The listing builds one solid part. Answer for the finished solid, in the listing's coordinates (mm). A direction names the side the tool comes from. Coordinates: 2 decimals unless noted, no trailing zeros. Write each loop counter-clockwise with the first axis right and the second up, starting at its lowest first coordinate (ties: lowest second). Pieces come first, ordered by that corner, then holes.
```python
from build123d import *

# Parameters (mm, degrees)
SKETCH1_W           = 30
SKETCH1_H           = 30
BOSS_EXTRUDE2_DEPTH = 35
SKETCH2_W           = 25
SKETCH2_H           = 25
CUT_EXTRUDE1_DEPTH  = 10
SKETCH3_R           = 5
SKETCH3_R_2         = 2
CUT_EXTRUDE4_DEPTH  = 20
SKETCH5_R           = 2
CUT_EXTRUDE5_DEPTH  = 25


with BuildPart() as part:
    # Sketch1 → Boss-Extrude2 (new body)
    with BuildSketch(Plane(origin=(0, 0, 0), x_dir=(1, 0, 0), z_dir=(0, 1, 0))):
        Rectangle(SKETCH1_W, SKETCH1_H)
    extrude(amount=BOSS_EXTRUDE2_DEPTH)

    # Sketch2 → Cut-Extrude1 (cut)
    with BuildSketch(Plane(origin=(0, 35, 0), x_dir=(1, 0, 0), z_dir=(0, 1, 0))):
        with Locations((2.5, 2.5)):
            Rectangle(SKETCH2_W, SKETCH2_H)
    extrude(amount=-CUT_EXTRUDE1_DEPTH, mode=Mode.SUBTRACT)

    # Sketch3 → Cut-Extrude4 (cut)
    # profile 1 of 2: a face of its own
    with BuildSketch(Plane(origin=(0, 25, 0), x_dir=(1, 0, 0), z_dir=(0, 1, 0))):
        with Locations(Location((-2.422862762, 7.422862762, 0), (0, 0, 270))):
            Circle(SKETCH3_R)
        with Locations(Location((-2.422862762, 7.422862762, 0), (0, 0, 270))):
            Circle(SKETCH3_R_2, mode=Mode.SUBTRACT)
    # profile 2 of 2: a face of its own
    with BuildSketch(Plane(origin=(0, 25, 0), x_dir=(1, 0, 0), z_dir=(0, 1, 0))):
        with Locations(Location((8.75, -3.75, 0), (0, 0, 270))):
            Circle(SKETCH3_R)
        with Locations(Location((8.75, -3.75, 0), (0, 0, 270))):
            Circle(SKETCH3_R_2, mode=Mode.SUBTRACT)
    extrude(amount=-CUT_EXTRUDE4_DEPTH, mode=Mode.SUBTRACT)

    # Sketch5 → Cut-Extrude5 (cut)
    with BuildSketch(Plane(origin=(0, 25, 0), x_dir=(1, 0, 0), z_dir=(0, 1, 0))):
        with Locations(Location((-2.422862762, 7.422862762, 0), (0, 0, 270))):
            Circle(SKETCH5_R)
        with Locations(Location((8.75, -3.75, 0), (0, 0, 270))):
            Circle(SKETCH5_R)
    extrude(amount=-CUT_EXTRUDE5_DEPTH, mode=Mode.SUBTRACT)


solid = part.part
```
(1) Section A-A, the plane x = 8.75 is taken. Write down the section's boundary in (y, z).
(2) Section C-C, the plane y = 4 is taken. Write down the section's boundary in (x, z).
(3) Find the intervals of material crossed by probe 1 along X at (y, z) = (12.25, 3.75); probe 2 along Y at (x, z) = (1, -13.25); probe 3 along Z at (x, y) = (-7.5, 33.5), in increasing order.
(4) Section D-D, the plane z = -3.75 is taken. Write down the section's boundary in (x, y).
(5) Each of these flat-tipped pins is pushed along its axis until it touches: pin 1 (6 mm diameter, centred on x = 10, z = 9, fed in from +Y); pin 2 (4.5 mm diameter, centred on x = 8.75, z = 3.75, fed in from +Y); pin 3 (5 mm diameter, centred on y = 30, z = 1.5, fed in from +X); pin 4 (7.5 mm diameter, centred on x = -3.5, z = -3, fed in from +Y). Where does it stop, or does it pass through?
(6) Which of the six approach directions +Z, -Z, +X, -X, +Y, -Y give full straight-line access (tool end or side, diameter ignored) to faces 1 (the flat face through (-10, 30, -2)), 2 (the flat face through (-11, 35, 5)), 3 (the cylindrical face through (-5.465, 15.14, -11.391))?
(7) Section B-B, the plane z = 3.75 is taken. Write down the section's boundary in (x, y).
(8) For a pull along Z with two mould halves and no side action, classify faces 4 (the cylindrical face through (-3.64, 2.54, -9.01)), 5 (the flat face through (0, 17, 15)), 6 (the flat face through (2, 30, 10)) as pulls with the +Z half, pulls with the -Z half, needs draft (parallel to the pull), parting line crosses it, or undercut.
Solution:
1. outline: (0, -15) - (25, -15) - (25, -1.25) - (5, -1.25) - (5, 1.75) - (0, 1.75) - close; (0, 5.75) - (5, 5.75) - (5, 8.75) - (25, 8.75) - (25, 10) - (35, 10) - (35, 15) - (0, 15) - close
2. outline: (-15, -15) - (15, -15) - (15, 15) - (-15, 15) - close; hole circle Ø4 at (-2.42, -7.42); hole circle Ø4 at (8.75, 3.75)
3. probe 1: x = -15 to 3.75, 13.75 to 15
3. probe 2: y = 0 to 25
3. probe 3: z = 10 to 15
4. outline: (-15, 0) - (15, 0) - (15, 25) - (0.97, 25) - (0.97, 5) - (-5.82, 5) - (-5.82, 25) - (-10, 25) - (-10, 35) - (-15, 35) - close
5. pin 1: stops at y = 35
5. pin 2: stops at y = 5
5. pin 3: stops at x = -10
5. pin 4: stops at y = 25
6. face 1: -Z, +X, +Y
6. face 2: +Z, -Z, +X, -X, +Y
6. face 3: +Y
7. outline: (-15, 0) - (6.75, 0) - (6.75, 5) - (3.75, 5) - (3.75, 25) - (-10, 25) - (-10, 35) - (-15, 35) - close; (10.75, 0) - (15, 0) - (15, 25) - (13.75, 25) - (13.75, 5) - (10.75, 5) - close
8. face 4: undercut
8. face 5: pulls with the +Z half
8. face 6: pulls with the -Z half
